For this review, take the finished solid that the model builds, in its own axes (mm). A direction names the side the tool comes from. Give positions to 0.01 mm unless a question says otherwise; leave off trailing zeros. Loops run counter-clockwise (first coordinate to the right, second up) from the corner with the lowest first, then second, coordinate; pieces in that order, holes last. Notation, with made-up numbers: (33, -0.5) - (54, -0.5) arc R20 ccw to (54, 11.5) - close; hole circle Ø3 at (1, -29.75). An arc over 180 degrees is marked (long way). Answer as CSV lines item,"result".
from build123d import *

# Parameters (mm, degrees)
BOSS_EXTRUDE1_DEPTH = 208.295833
SKETCH3_R           = 77.5
CUT_EXTRUDE1_DEPTH  = 145


with BuildPart() as part:
    # Sketch2 → Boss-Extrude1 (new body)
    with BuildSketch(Plane.XY.offset(2)):
        Polygon((9824.878184452, 584.852821259), (9909.787083093, 615.730562922), (9909.905272796, 610.453189538), (9826.586986697, 580.153885753), align=None)
    extrude(amount=BOSS_EXTRUDE1_DEPTH)

    # Sketch3 → Cut-Extrude1 (cut)
    with BuildSketch(Plane.XY.offset(156.31)):
        with Locations((9942.206448064, 615.592583884)):
            Circle(SKETCH3_R)
    extrude(amount=-CUT_EXTRUDE1_DEPTH, mode=Mode.SUBTRACT)


solid = part.part
1) Consider section A-A on y = 603. Write out the cut boundary in (x, z).
From the geometry:
outline,"(9874.78, 2) - (9889.41, 2) - (9889.41, 11.31) - (9874.78, 11.31) - close; (9874.78, 156.31) - (9889.41, 156.31) - (9889.41, 210.3) - (9874.78, 210.3) - close"
2) Consider section C-C on z = 171. Write out the cut boundary in (x, y), and give its area (3 significant figures).
From the geometry:
outline,"(9824.88, 584.85) - (9826.59, 580.15) - (9909.91, 610.45) - (9909.79, 615.73) - close"
area,"448 mm^2"
3) Consider section D-D on x = 9861. Write out the cut boundary in (y, z), and give its area (3 significant figures).
From the geometry:
outline,"(592.67, 2) - (597.99, 2) - (597.99, 210.3) - (592.67, 210.3) - close"
area,"1,110 mm^2"
4) Insertion check: P1, Ø1.5, axis at x = 9856, z = 177, coming from the -Y side; P2, Ø1.5, axis at x = 9841.5, z = 147.5, coming from the +Y side; P3, Ø8, axis at y = 604.5, z = 125.5, coming from the -X side. Each pin has a flat end and moves straight along its axis. Give the tip position at first contact, or say it passes through.
From the geometry:
P1,"stops at y = 590.58"
P2,"stops at y = 591.17"
P3,"passes through"
5) Machinability: for faces 5 (the flat face through (9847.87, 593.214, 127.834)), 6 (the cylindrical face through (9866.848, 597.498, 84.825)), which of the approach directions +Z, -Z, +X, -X, +Y, -Y give a long, thin tool a straight path to every point of the face, cutting with its end or side? Answer none if there is none.
From the geometry:
face 5,"+Z, -Z, -X, +Y"
face 6,"+X, +Y"
6) Consider section B-B on x = 9898. Write out the cut boundary in (y, z), and give its area (3 significant figures).
From the geometry:
outline,"(606.12, 2) - (611.44, 2) - (611.44, 11.31) - (606.12, 11.31) - close; (606.12, 156.31) - (611.44, 156.31) - (611.44, 210.3) - (606.12, 210.3) - close"
area,"337 mm^2"
7) Draft analysis for pull direction Z (two halves, no side actions). For faces 1 (the flat face through (9850.31, 588.78, 127.83)), 2 (the flat face through (9888, 605, 11.31)), 3 (the flat face through (9868, 598, 2)), 4 (the flat face through (9868, 598, 210.296)), state which applies: pulls with the +Z half, pulls with the -Z half, needs draft (parallel to the pull), parting line crosses it, or undercut.
From the geometry:
face 1,"needs draft"
face 2,"undercut"
face 3,"pulls with the -Z half"
face 4,"pulls with the +Z half"
8) Wall thickness on line 1 (Z direction, x = 9886.5, y = 606); line 2 (Y direction, x = 9858, z = 181.5); line 3 (Y direction, x = 9848, z = 25): over which ranges is each line inside the solid? List them lowest first. Write a range as from..to.
From the geometry:
line 1,"z = 2..11.31, 156.31..210.3"
line 2,"y = 591.58..596.9"
line 3,"y = 587.94..593.26"
